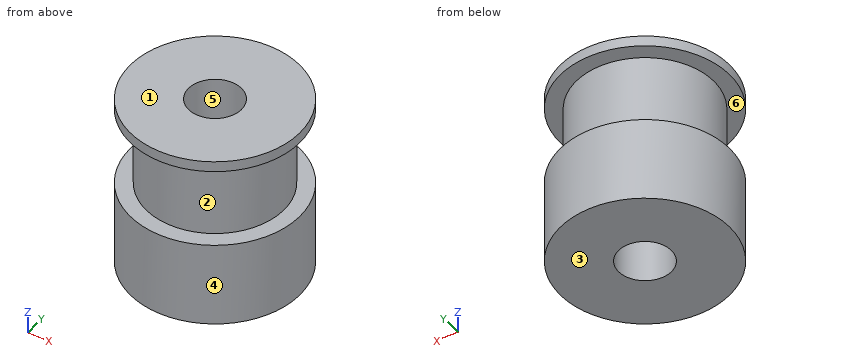
Autodesk Inventor part; units mm, degrees
ref_plane "YZ Plane" through (0, 0, 0) normal (1, 0, 0) x (0, 1, 0)
ref_plane "XZ Plane" through (0, 0, 0) normal (0, 1, 0) x (-1, 0, 0)
ref_plane "XY Plane" through (0, 0, 0) normal (0, 0, 1) x (1, 0, 0)
sketch "Szkic1" plane through (0, 0, 0) normal (0, 0, 1) x (1, 0, 0)
  circle A0 centre (0, 0) radius 2.5
  circle A1 centre (0, 0) radius 8
  dimension "d0" = 5
  dimension "d1" = 16
extrude "Wyciągnięcie proste1" add sketch "Szkic1" along normal blind 8
sketch "Szkic2" plane through (0, 0, 8) normal (0, 0, 1) x (1, 0, 0)
  circle A0 centre (0, 0) radius 2.5
  circle A1 centre (0, 0) radius 8
  circle A2 centre (0, 0) radius 6.5
  dimension "d4" = 13
extrude "Wyciągnięcie proste2" add sketch "Szkic2" along normal blind 7.5 contours A2
sketch "Szkic3" plane through (0, 0, 15.5) normal (0, 0, 1) x (1, 0, 0)
  circle A0 centre (0, 0) radius 6.5
  circle A1 centre (0, 0) radius 8
  circle A2 centre (0, 0) radius 2.5
  circle A3 centre (0, 0) radius 6.5
extrude "Wyciągnięcie proste3" add sketch "Szkic3" along normal blind 1 contours A0 | A1
properties part number "COTS_GENERIC_MXL_Pulley_X_Axis"
The model under review builds one solid part; all positions refer to its coordinate system, in mm. Face numbers are marked on the shaded views. A direction names the side the tool comes from. Coordinates: 2 decimals unless noted, no trailing zeros. Loops run counter-clockwise (first coordinate to the right, second up) from the corner with the lowest first, then second, coordinate; pieces in that order, holes last. Notation, with made-up numbers: (15, 35.25) -> (53, 35.25) arc R18 ccw to (53, 50.25) -> close; hole circle Ø1 at (1, -27.75). An arc over 180 degrees is marked (long way). Use a Markdown table: item, result. Add a question column.
1. To check wall thickness, follow line 1 (Y direction, x = 0, z = 8.75); line 2 (Z direction, x = -6.75, y = -1); line 3 (X direction, y = -1.5, z = 2.25). State the ranges of each line that lie inside material, in increasing order.
2. Clearance check with flat-ended pins moving along their axes: pin 1 Ø3 at (x, z) = (2, 14.5) entering from +Y; pin 2 Ø3 at (x, z) = (-2.5, 4.5) entering from -Y; pin 3 Ø1 at (y, z) = (6, 9) entering from +X. State where each tip first meets the part, or that it passes through.
3. Machinability: for the marked faces 5 and 6, which of the approach directions +Z, -Z, +X, -X, +Y, -Y give a long, thin tool a straight path to every point of the face, cutting with its end or side? Answer none if there is none.
4. Add section C-C on y = 5.25. Write out the cut boundary in (x, z).
5. Add section D-D on x = 3.5. Write out the cut boundary in (y, z), plus the area to 3 significant figures.
6. Add section A-A on y = 0. Write out the cut boundary in (x, z), plus the area to 3 significant figures.
7. Draft analysis for pull direction Z (two halves, no side actions). For the marked faces 1, 2, 3 and 4, state which applies: pulls with the +Z half, pulls with the -Z half, needs draft (parallel to the pull), parting line crosses it, or undercut.
Returned:
| question | item | result |
|---|---|---|
| 1 | line 1 | y = -6.5 to -2.5, 2.5 to 6.5 |
| 1 | line 2 | z = 0 to 8, 15.5 to 16.5 |
| 1 | line 3 | x = -7.86 to -2, 2 to 7.86 |
| 2 | pin 1 | stops at y = 7.95 |
| 2 | pin 2 | stops at y = -7.94 |
| 2 | pin 3 | stops at x = 3.46 |
| 3 | face 5 | +Z, -Z |
| 3 | face 6 | none |
| 4 | outline | (-6.04, 0) -> (6.04, 0) -> (6.04, 8) -> (3.83, 8) -> (3.83, 15.5) -> (6.04, 15.5) -> (6.04, 16.5) -> (-6.04, 16.5) -> (-6.04, 15.5) -> (-3.83, 15.5) -> (-3.83, 8) -> (-6.04, 8) -> close |
| 5 | outline | (-7.19, 0) -> (7.19, 0) -> (7.19, 8) -> (5.48, 8) -> (5.48, 15.5) -> (7.19, 15.5) -> (7.19, 16.5) -> (-7.19, 16.5) -> (-7.19, 15.5) -> (-5.48, 15.5) -> (-5.48, 8) -> (-7.19, 8) -> close |
| 5 | area | 212 mm² |
| 6 | outline | (-8, 0) -> (-2.5, 0) -> (-2.5, 16.5) -> (-8, 16.5) -> (-8, 15.5) -> (-6.5, 15.5) -> (-6.5, 8) -> (-8, 8) -> close; (2.5, 0) -> (8, 0) -> (8, 8) -> (6.5, 8) -> (6.5, 15.5) -> (8, 15.5) -> (8, 16.5) -> (2.5, 16.5) -> close |
| 6 | area | 159 mm² |
| 7 | face 1 | pulls with the +Z half |
| 7 | face 2 | undercut |
| 7 | face 3 | pulls with the -Z half |
| 7 | face 4 | needs draft |
